Part model, mm, in its own coordinate system. A direction names the side the tool comes from. Give positions to 0.01 mm unless a question says otherwise; leave off trailing zeros. Order: outer loops, then holes, each group sorted by start corner. A loop starts at its lowest first (then second) coordinate and runs counter-clockwise, first axis right, second up.
1. Slice it at A-A on z = 28. List the corners of the cut face in (x, y).
2. Which spindle directions (+Z, -Z, +X, -X, +Y, -Y) get a long thin tool onto all of the face, cutting with end or side? Do faces 5 (the flat face through (12.168, -20.688, 5.916)), 6 (the cylindrical face through (-1.08, -4.88, 28.54)), 7 (the flat face through (11, -12, 12)). Say none if no direction does.
3. Mould opens along Y. For faces 1 (the cylindrical face through (11.923, 3.755, 31.07)), 2 (the flat face through (-0.1, -3.3, 31)), 3 (the cylindrical face through (13.267, -12.165, 25.647)), 4 (the flat face through (0, 0, 0)) say: +Y half, -Y half, draft (parallel to the pull), parting line (faces both ways), or undercut.
4. Probe line 1 (Y direction, x = 0, z = 27.8); line 2 (Y direction, x = 0, z = 33); line 3 (Z direction, x = -11, y = 12). List the from-to ranges inside material, lowest first.
5. Slice it at B-B on y = 0. List the corners of the cut face in (x, z), and give its area (3 significant figures).
6. Drop flat-ended pins along their axis: pin 1 Ø10 at (x, y) = (14, -15.5) entering from +Z; pin 2 Ø8 at (x, y) = (1, -2.5) entering from +Z; pin 3 Ø5 at (x, z) = (1.5, 26) entering from +Y; pin 4 Ø3 at (x, z) = (-6.5, 30.5) entering from +Y. Give the stop position or say it passes through.
7. Slice it at C-C on z = 4. List the corners of the cut face in (x, y).
8. Slice it at D-D on x = -8.5. List the corners of the cut face in (y, z), and give its area (3 significant figures).
from build123d import *

# Parameters (mm, degrees)
SKETCH_2_R          = 12.5
SKETCH_2_R_2        = 5
CUT_EXTRUDE_1_DEPTH = 10
SKETCH_3_R          = 3
CUT_EXTRUDE_2_DEPTH = 10
SKETCH_4_R          = 5
CUT_EXTRUDE_3_DEPTH = 5
EXTRUDE_1_DEPTH     = 12


with BuildPart() as part:
    # 草图1 → 旋转1 (revolve)
    with BuildSketch(Plane(origin=(0, 0, 0), x_dir=(0, 0, -1), z_dir=(1, 0, 0)), mode=Mode.PRIVATE) as revolve_1_sk:
        Polygon((0, 0), (0, 24), (-12, 24), (-12, 16), (-15, 16), (-15, 18), (-36, 18), (-36, 0), align=None)
    revolve(revolve_1_sk.sketch.rotate(Axis((0, 0, 0), (0, 0, 1)), 90), axis=Axis((0, 0, 0), (0, 0, 1)))

    # 草图2 → 切除-拉伸1 (cut)
    with BuildSketch(Plane.XY.offset(36)):
        Circle(SKETCH_2_R)
        Circle(SKETCH_2_R_2, mode=Mode.SUBTRACT)
    extrude(amount=-CUT_EXTRUDE_1_DEPTH, mode=Mode.SUBTRACT)

    # 草图3 → 切除-拉伸2 (cut)
    with BuildSketch(Plane.XY.offset(36)):
        Circle(SKETCH_3_R)
    extrude(amount=-CUT_EXTRUDE_2_DEPTH, mode=Mode.SUBTRACT)

    # 草图4 → 切除-拉伸3 (cut)
    with BuildSketch(Plane.XY.offset(36)):
        Circle(SKETCH_4_R)
    extrude(amount=-CUT_EXTRUDE_3_DEPTH, mode=Mode.SUBTRACT)

    # 草图5 → 凸台-拉伸1 (add)
    with BuildSketch(Plane(origin=(0, 0, 0), x_dir=(-1, 0, 0), z_dir=(0, 0, -1))):
        Polygon((0, 27.712812921), (-24, 13.856406461), (-24, -13.856406461), (0, -27.712812921), (24, -13.856406461), (24, 13.856406461), align=None)
    extrude(amount=-EXTRUDE_1_DEPTH)


solid = part.part
Data:
1. outline: circle Ø36 at (0, 0); circle Ø10 at (0, 0); hole circle Ø25 at (0, 0); hole circle Ø6 at (0, 0)
2. face 5: +Z, -Z, +X, -Y
2. face 6: +Z
2. face 7: none
3. face 1: undercut
3. face 2: undercut
3. face 3: parting line
3. face 4: draft
4. line 1: y = -18 to -12.5, -5 to -3, 3 to 5, 12.5 to 18
4. line 2: y = -18 to -12.5, 12.5 to 18
4. line 3: z = 0 to 12, 15 to 36
5. outline: (-24, 0) - (24, 0) - (24, 12) - (16, 12) - (16, 15) - (18, 15) - (18, 36) - (12.5, 36) - (12.5, 26) - (5, 26) - (5, 31) - (3, 31) - (3, 26) - (-3, 26) - (-3, 31) - (-5, 31) - (-5, 26) - (-12.5, 26) - (-12.5, 36) - (-18, 36) - (-18, 15) - (-16, 15) - (-16, 12) - (-24, 12) - close
5. area: 1,200 mm2
6. pin 1: stops at z = 36
6. pin 2: stops at z = 31
6. pin 3: stops at y = 18
6. pin 4: stops at y = 17.29
7. outline: (-24, -13.86) - (0, -27.71) - (24, -13.86) - (24, 13.86) - (0, 27.71) - (-24, 13.86) - close
8. outline: (-22.81, 0) - (22.81, 0) - (22.81, 12) - (13.56, 12) - (13.56, 15) - (15.87, 15) - (15.87, 36) - (9.17, 36) - (9.17, 26) - (-9.17, 26) - (-9.17, 36) - (-15.87, 36) - (-15.87, 15) - (-13.56, 15) - (-13.56, 12) - (-22.81, 12) - close
8. area: 1,110 mm2
